Source: CAD feature listing. Evaluate the final solid. Frame: model axes, mm. Face numbers are marked on the shaded views. A direction names the side the tool comes from. Give positions to 0.01 mm unless a question says otherwise; leave off trailing zeros. Order: outer loops, then holes, each group sorted by start corner. A loop starts at its lowest first (then second) coordinate and runs counter-clockwise, first axis right, second up.
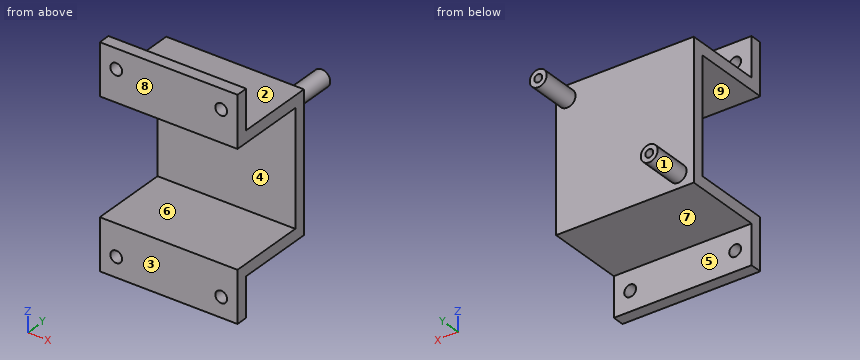
from build123d import *

# Parameters (mm, degrees)
SKETCH1_W           = 35
SKETCH1_H           = 35
BOSS_EXTRUDE1_DEPTH = 3
SKETCH2_R           = 2.15
SKETCH2_R_2         = 1
BOSS_EXTRUDE2_DEPTH = 10
SKETCH3_W           = 35
SKETCH3_H           = 3
BOSS_EXTRUDE3_DEPTH = 20
SKETCH4_W           = 35
SKETCH4_H           = 3
BOSS_EXTRUDE4_DEPTH = 10
SKETCH5_R           = 1.5
CUT_EXTRUDE1_DEPTH  = 10


with BuildPart() as part:
    # Sketch1 → Boss-Extrude1 (new body)
    with BuildSketch(Plane(origin=(0, 0, 0), x_dir=(1, 0, 0), z_dir=(0, 1, 0))):
        Rectangle(SKETCH1_W, SKETCH1_H)
    extrude(amount=BOSS_EXTRUDE1_DEPTH)

    # Sketch2 → Boss-Extrude2 (add)
    # profile 1 of 2: a face of its own
    with BuildSketch(Plane(origin=(0, 3, 0), x_dir=(1, 0, 0), z_dir=(0, 1, 0))):
        with Locations(Location((-13.512690171, 13.984805963, 0), (0, 0, 90))):
            Circle(SKETCH2_R)
        with Locations(Location((-13.512690171, 13.984805963, 0), (0, 0, 270))):
            Circle(SKETCH2_R_2, mode=Mode.SUBTRACT)
    # profile 2 of 2: a face of its own
    with BuildSketch(Plane(origin=(0, 3, 0), x_dir=(1, 0, 0), z_dir=(0, 1, 0))):
        with Locations(Location((14.687309829, -14.215194037, 0), (0, 0, 90))):
            Circle(SKETCH2_R)
        with Locations(Location((14.687309829, -14.215194037, 0), (0, 0, 270))):
            Circle(SKETCH2_R_2, mode=Mode.SUBTRACT)
    extrude(amount=BOSS_EXTRUDE2_DEPTH)

    # Sketch3 → Boss-Extrude3 (add)
    with BuildSketch(Plane.XZ):
        with Locations((0, 16)):
            Rectangle(SKETCH3_W, SKETCH3_H)
        with Locations((0, -16)):
            Rectangle(SKETCH3_W, SKETCH3_H)
    extrude(amount=BOSS_EXTRUDE3_DEPTH)

    # Sketch4 → Boss-Extrude4 (add)
    with BuildSketch(Plane(origin=(0, 0, -17.5), x_dir=(-1, 0, 0), z_dir=(0, 0, -1))):
        with Locations((0, -18.5)):
            Rectangle(SKETCH4_W, SKETCH4_H)
    boss_extrude4 = extrude(amount=BOSS_EXTRUDE4_DEPTH)

    # Sketch5 → Cut-Extrude1 (cut)
    with BuildSketch(Plane(origin=(0, -17, 0), x_dir=(1, 0, 0), z_dir=(0, 1, 0))):
        with Locations(Location((-13.324621587, 22.5, 0), (0, 0, 180))):
            Circle(SKETCH5_R)
        with Locations(Location((13.355252901, 22.5, 0), (0, 0, 180))):
            Circle(SKETCH5_R)
    cut_extrude1 = extrude(amount=-CUT_EXTRUDE1_DEPTH, mode=Mode.SUBTRACT)

    # Mirror1: Boss-Extrude4, Cut-Extrude1 across plane
    add(boss_extrude4.mirror(Plane.XY))
    add(cut_extrude1.mirror(Plane.XY), mode=Mode.SUBTRACT)


solid = part.part
1) Ray query, L1, parallel to X at y = -18.5, z = 22.5; L2, parallel to Z at x = 7.5, y = -6; L3, parallel to Y at x = 0.5, z = -11. Return the intervals inside material, ascending.
Checks:
L1: x = -17.5 to -14.82, -11.82 to 11.86, 14.86 to 17.5
L2: z = -17.5 to -14.5, 14.5 to 17.5
L3: y = 0 to 3
2) Section query B-B on y = -9.5. Output: boundary loops of the cut face in (x, z).
Checks:
outline: (-17.5, -17.5) - (17.5, -17.5) - (17.5, -14.5) - (-17.5, -14.5) - close; (-17.5, 14.5) - (17.5, 14.5) - (17.5, 17.5) - (-17.5, 17.5) - close
3) Pull-direction query (Z, two-part tool) for the marked faces 6, 7, 8 and 9; classes: +Z half, -Z half, draft (parallel to the pull), parting line (faces both ways), or undercut.
Checks:
face 6: undercut
face 7: -Z half
face 8: draft
face 9: undercut
4) Section query A-A on z = 22.5. Output: boundary loops of the cut face in (x, y).
Checks:
outline: (-17.5, -20) - (-14.82, -20) - (-14.82, -17) - (-17.5, -17) - close; (-11.82, -20) - (11.86, -20) - (11.86, -17) - (-11.82, -17) - close; (14.86, -20) - (17.5, -20) - (17.5, -17) - (14.86, -17) - close
5) Reachability of the marked faces 1, 2, 3, 4 and 5 from +Z, -Z, +X, -X, +Y, -Y: full face, straight path, thin tool, end or side. Return the list, or none.
Checks:
face 1: +Y
face 2: +Z, +X, -X, +Y
face 3: +Z, -Z, +X, -X, -Y
face 4: +X, -X, -Y
face 5: -Z, +X, -X, +Y
6) Section query D-D on x = -7. Output: boundary loops of the cut face in (y, z), and give its area (3 significant figures).
Checks:
outline: (-20, -27.5) - (-17, -27.5) - (-17, -17.5) - (3, -17.5) - (3, 17.5) - (-17, 17.5) - (-17, 27.5) - (-20, 27.5) - (-20, 14.5) - (0, 14.5) - (0, -14.5) - (-20, -14.5) - close
area: 285 mm2
7) First-contact query: pin 1 Ø17.5 at (x, z) = (5.5, -8.5) entering from +Y; pin 2 Ø10 at (x, y) = (-4, -7.5) entering from -Z; pin 3 Ø3 at (y, z) = (4, 16) entering from +X; pin 4 Ø6 at (x, y) = (-7.5, -10.5) entering from +Z. Flat tips, straight axial feed; report the tip coordinate or a pass-through.
Checks:
pin 1: stops at y = 3
pin 2: stops at z = -17.5
pin 3: stops at x = 17.5
pin 4: stops at z = 17.5
8) Section query C-C on y = 8. Output: boundary loops of the cut face in (x, z).
Checks:
outline: circle Ø4.3 at (-13.51, -13.98); circle Ø4.3 at (14.69, 14.22); hole circle Ø2 at (-13.51, -13.98); hole circle Ø2 at (14.69, 14.22)
